For this review, use the dimensioned drawing (mm, ordinates from the lowest corner) and the shaded views. A direction names the side the tool comes from. Round coordinates to 2 decimals unless told otherwise and drop trailing zeros. Write each loop counter-clockwise with the first axis right and the second up, starting at its lowest first coordinate (ties: lowest second). Pieces come first, ordered by that corner, then holes. Notation, with made-up numbers: M -19.75,43 L 20.25,43 A33 cw 20.25,81 Z; hole C 17.5,27.5 d4. An arc over 180 degrees is marked long. Use one line per item in the form item = value. Start each with the question number.
Item 1: Add section D-D (y = 23). State the section outline as (x, z) points.
Item 2: Add section C-C (x = 50). State the section outline as (y, z) points, and give its area (3 significant figures).
Item 3: For P1, Ø2, axis at x = 68.5, z = 10.5, coming from the -Y side; P2, Ø3, axis at x = 34.5, z = 6, coming from the -Y side; P3, Ø6, axis at x = 53.5, y = 6.5, coming from the -Z side, all flat-tipped, find the tip position at first contact; note any pin that passes through.
Item 4: Add section B-B (z = 12). State the section outline as (x, y) points, and give its area (3 significant figures).
Item 5: For line 1 (Z direction, x = 50, y = 26.45); line 2 (X direction, y = 27.4, z = 12); line 3 (X direction, y = 20.75, z = 8.25), list the stretches that pass through material, from the lowest coordinate up. Write a range as [from, to].
Item 6: For the marked faces 1, 2 and 3, list the 3-axis set-ups (+Z, -Z, +X, -X, +Y, -Y) from which the entire face can be reached by the end or side of a thin tool; tool diameter is ignored.
Item 7: Add section A-A (y = 27.5). State the section outline as (x, z) points, and give its area (3 significant figures).
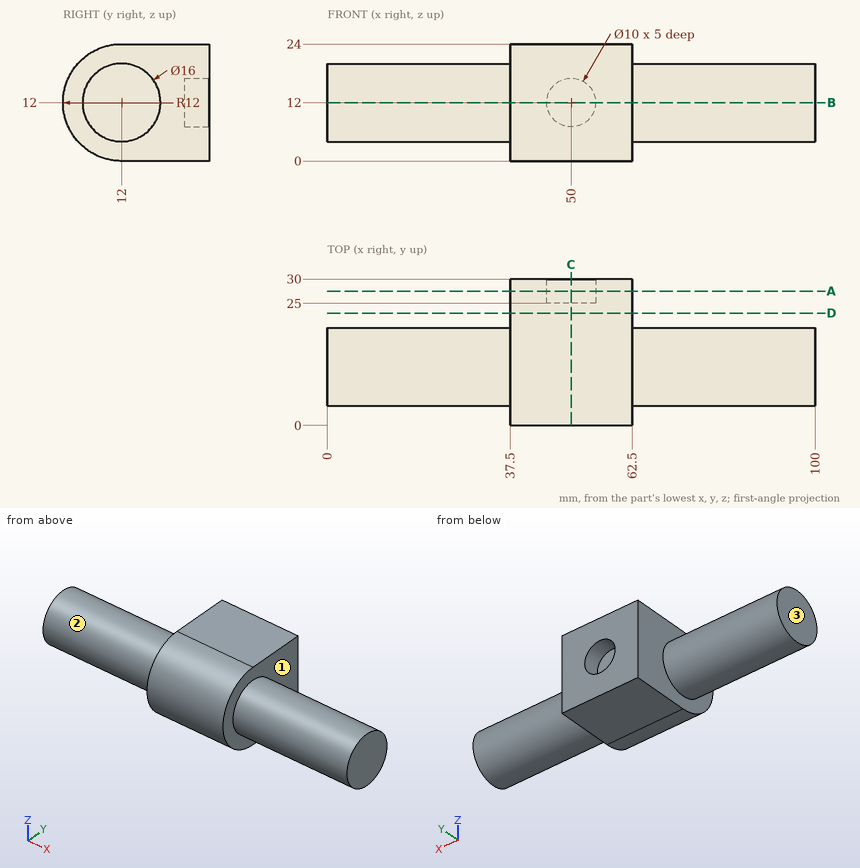
Calculated:
q1.outline = M 37.5,0 L 62.5,0 L 62.5,24 L 37.5,24 Z
q2.outline = M 12,0 L 30,0 L 30,7 L 25,7 L 25,17 L 30,17 L 30,24 L 12,24 A12 ccw Z
q2.area = 608 mm^2
q3.P1 = 4.02
q3.P2 = 5.39
q3.P3 = 0.26
q4.outline = M 0,4 L 37.5,4 L 37.5,0 L 62.5,0 L 62.5,4 L 100,4 L 100,20 L 62.5,20 L 62.5,30 L 55,30 L 55,25 L 45,25 L 45,30 L 37.5,30 L 37.5,20 L 0,20 Z
q4.area = 1,900 mm^2
q5.line_1 = [0, 7], [17, 24]
q5.line_2 = [37.5, 45], [55, 62.5]
q5.line_3 = [37.5, 62.5]
q6.face_1 = +X
q6.face_2 = -X
q6.face_3 = +Z, -Z, -X, +Y, -Y
q7.outline = M 37.5,0 L 62.5,0 L 62.5,24 L 37.5,24 Z; hole C 50,12 d10
q7.area = 521 mm^2
